```python
from build123d import *

# Parameters (mm, degrees)
F1_DEPTH = 25.4
F3_DEPTH = 25.4
F4_R     = 6.35
F5_DEPTH = 127
F7_DEPTH = 25.4
F9_DEPTH = 25.4


# Not quite as in the source:
# - a feature names something its author has since deleted; it is built from what else it names


with BuildPart() as f1:
    # F0 (on Front) → F1 (new body)
    with BuildSketch(Plane.XZ):
        Polygon((-28.758216656, 38.1), (-54.158216656, 38.1), (-54.158216656, 0), (22.041783344, 0), (22.041783344, 12.7), (-28.758216656, 12.7), align=None)
    extrude(amount=F1_DEPTH)

    # F2 (on face) → F3 (join)
    with BuildSketch(Plane.XY.offset(12.7)):
        with BuildLine():
            Line((-28.758216656, 0), (-28.758216656, -25.4))
            ThreePointArc((-28.758216656, -25.4), (-23.817550475, -12.7), (-28.758216656, 0))
        make_face()
    extrude(amount=F3_DEPTH)

    # F4 (on face) → F5 (cut)
    with BuildSketch(Plane.XY.offset(38.1)):
        with BuildLine():
            ThreePointArc((-54.158216656, -12.7), (-50.438472777, -3.7197438789), (-41.458216656, 0))
            Line((-41.458216656, 0), (-54.158216656, 0))
            Line((-54.158216656, 0), (-54.158216656, -12.7))
        make_face()
        with BuildLine():
            Line((-54.158216656, -25.4), (-41.458216656, -25.4))
            ThreePointArc((-41.458216656, -25.4), (-50.438472777, -21.6802561211), (-54.158216656, -12.7))
            Line((-54.158216656, -12.7), (-54.158216656, -25.4))
        make_face()
        with Locations((-41.458216656, -12.7)):
            Circle(F4_R)
    extrude(amount=-F5_DEPTH, mode=Mode.SUBTRACT)

    # F6 (on face) → F7 (cut)
    with BuildSketch(Plane.XY.offset(38.1)):
        with BuildLine():
            ThreePointArc((-37.5933498144, 0), (-28.6296169388, -12.9065923281), (-38.1607972085, -25.4))
            Line((-38.1607972085, -25.4), (-28.758216656, -25.4))
            ThreePointArc((-28.758216656, -25.4), (-23.817550475, -12.7), (-28.758216656, 0))
            Line((-28.758216656, 0), (-37.5933498144, 0))
        make_face()
    extrude(amount=-F7_DEPTH, mode=Mode.SUBTRACT)

    # F8 (on face) → F9 (cut)
    with BuildSketch(Plane.XY.offset(12.7)):
        with BuildLine():
            ThreePointArc((15.691783344, -12.7), (13.8319114046, -8.2098719395), (9.341783344, -6.35))
            ThreePointArc((9.341783344, -6.35), (2.991783344, -12.7), (9.341783344, -19.05))
            ThreePointArc((9.341783344, -19.05), (13.8319114046, -17.1901280605), (15.691783344, -12.7))
        make_face()
        with BuildLine():
            ThreePointArc((-15.9312973803, -6.35), (-11.4411693197, -8.2098719395), (-9.5812973803, -12.7))
            ThreePointArc((-9.5812973803, -12.7), (-11.4411693197, -17.1901280605), (-15.9312973803, -19.05))
            Line((-15.9312973803, -19.05), (9.341783344, -19.05))
            ThreePointArc((9.341783344, -19.05), (2.991783344, -12.7), (9.341783344, -6.35))
            Line((9.341783344, -6.35), (-15.9312973803, -6.35))
        make_face()
        with BuildLine():
            ThreePointArc((-15.9312973803, -19.05), (-11.4411693197, -17.1901280605), (-9.5812973803, -12.7))
            ThreePointArc((-9.5812973803, -12.7), (-11.4411693197, -8.2098719395), (-15.9312973803, -6.35))
            ThreePointArc((-15.9312973803, -6.35), (-22.2812973803, -12.7), (-15.9312973803, -19.05))
        make_face()
        with BuildLine():
            ThreePointArc((9.341783344, 0), (18.3220394651, -3.7197438789), (22.041783344, -12.7))
            Line((22.041783344, -12.7), (22.041783344, 0))
            Line((22.041783344, 0), (9.341783344, 0))
        make_face()
        with BuildLine():
            ThreePointArc((22.041783344, -12.7), (18.3220394651, -21.6802561211), (9.341783344, -25.4))
            Line((9.341783344, -25.4), (22.041783344, -25.4))
            Line((22.041783344, -25.4), (22.041783344, -12.7))
        make_face()
    extrude(amount=-F9_DEPTH, mode=Mode.SUBTRACT)


solid = f1.part
```
Geometry check sheet. Reference: the model listing, model coordinates, mm. A direction names the side the tool comes from. Coordinates: 2 decimals unless noted, no trailing zeros. Loops run counter-clockwise (first coordinate to the right, second up) from the corner with the lowest first, then second, coordinate; pieces in that order, holes last.
Item 1: Sectioned sample at B-B, the plane z = 8.5. Record the boundary of the cut face in (x, y).
Item 2: Thickness scan on line 1 (X direction, y = -16.75, z = 10); line 2 (X direction, y = -13.25, z = 7); line 3 (Z direction, x = -25, y = -17.25). Record the ranges inside material, lowest first.
Item 3: Access from +Z, -Z, +X, -X, +Y, -Y to the whole of each face (thin tool, end or side, straight path). Record for faces 1 (the face through (-44.4, -6.9, 38.1)), 2 (the face through (-28.626, -12.671, 25.578)), 3 (the face through (-3, -6.35, 6)).
Item 4: Sectioned sample at C-C, the plane y = -9.25. Record the boundary of the cut face in (x, z).
Item 5: Go/stop test with flat-tipped pins: pin 1 Ø1 at (y, z) = (-11.5, 27) entering from +X; pin 2 Ø4 at (x, y) = (-26.5, -3) entering from +Z. Record where each tip stops, or that it passes through.
Item 6: Sectioned sample at D-D, the plane x = -25. Record the boundary of the cut face in (y, z).
Item 7: Release check for a two-part mould opening along Y. For faces 4 (the face through (-25, -13, 0)), 5 (the face through (-35.59, -15.13, 19.32)), 6 (the face through (-22.28, -12.56, 6.44)), 7 (the face through (-22, -25.4, 11)) record: released by +Y, released by -Y, zero draft, split by the parting line, or undercut.
Item 8: Sectioned sample at A-A, the plane x = -15. Record the boundary of the cut face in (y, z), then the cut area to 3 significant figures.
Check result:
1. outline: (-41.46, -25.4) - (9.34, -25.4) arc R12.7 ccw to (9.34, 0) - (-41.46, 0) arc R12.7 ccw to start; hole circle Ø12.7 at (-41.46, -12.7); hole (-15.93, -19.05) - (9.34, -19.05) arc R6.35 ccw to (9.34, -6.35) - (-15.93, -6.35) arc R6.35 ccw to start
2. line 1: x = -53.5 to -46.35, -36.57 to -20.82, 14.23 to 21.38
2. line 2: x = -54.15 to -47.78, -35.13 to -22.26, 15.67 to 22.03
2. line 3: z = 0 to 12.7
3. face 1: +Z, +X, -X, +Y, -Y
3. face 2: +Z, +X
3. face 3: +Z, -Z
4. outline: (-53.68, 0) - (-46.79, 0) - (-46.79, 38.1) - (-53.68, 38.1) - close; (-36.13, 0) - (-21.26, 0) - (-21.26, 12.7) - (-29.06, 12.7) - (-29.06, 38.1) - (-36.13, 38.1) - close; (14.67, 0) - (21.56, 0) - (21.56, 12.7) - (14.67, 12.7) - close
5. pin 1: stops at x = -28.64
5. pin 2: stops at z = 12.7
6. outline: (-25.4, 0) - (0, 0) - (0, 12.7) - (-25.4, 12.7) - close
7. face 4: zero draft
7. face 5: undercut
7. face 6: undercut
7. face 7: released by -Y
8. outline: (-25.4, 0) - (-19.05, 0) - (-19.05, 12.7) - (-25.4, 12.7) - close; (-6.35, 0) - (0, 0) - (0, 12.7) - (-6.35, 12.7) - close
8. area: 161 mm2
